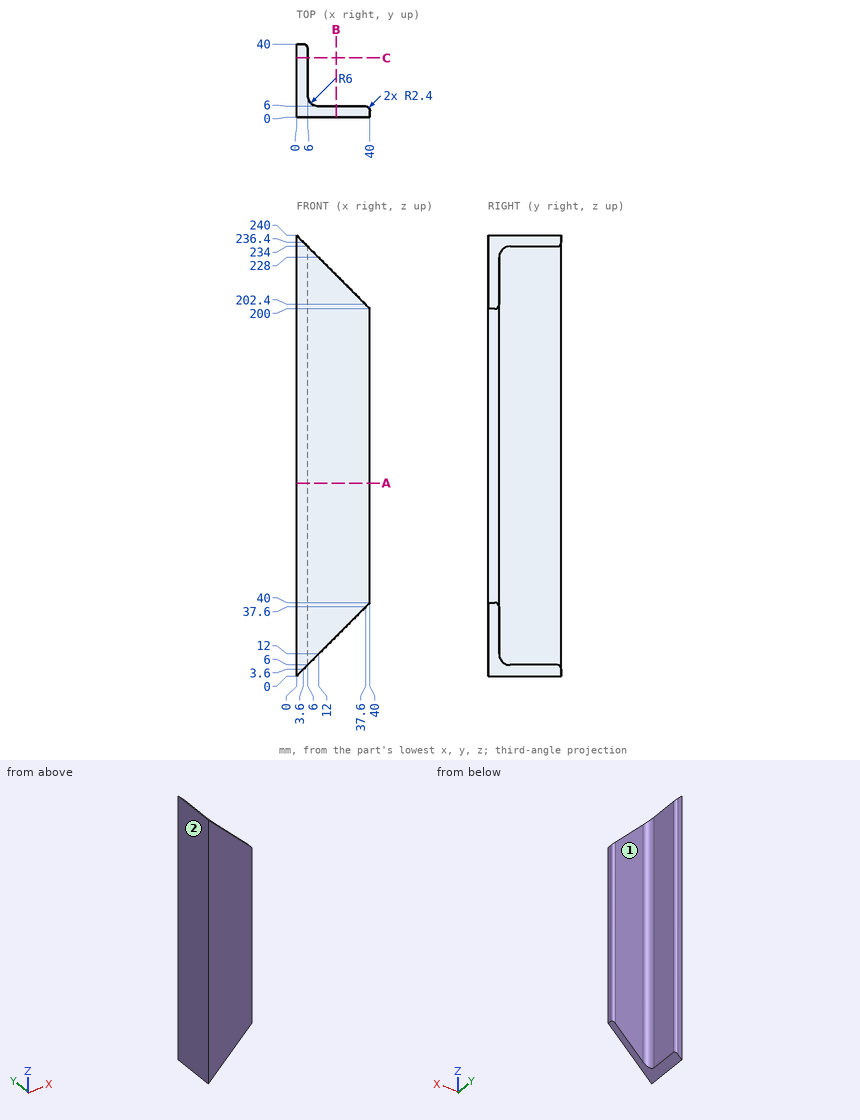
Job drawing, mm, ordinate dimensions from the low corner. One solid piece. A direction names the side the tool comes from. Coordinates: 2 decimals unless noted, no trailing zeros. Write each loop counter-clockwise with the first axis right and the second up, starting at its lowest first coordinate (ties: lowest second). Pieces come first, ordered by that corner, then holes.
Item 1: Slice it at A-A (z = 105). Write the cut outline in (x, y).
Item 2: Pin check, flat tips, straight feed: pin 1 (3 mm diameter, centred on x = 22.5, z = 57.5, fed in from +Y); pin 2 (2 mm diameter, centred on y = 35.5, z = 153, fed in from +X); pin 3 (12 mm diameter, centred on y = 10, z = 93.5, fed in from +X). Stop position of each tip, or through.
Item 3: Slice it at C-C (y = 32.5). Write the cut outline in (x, z).
Item 4: Probe line 1 (Y direction, x = 15.5, z = 143.5); line 2 (Y direction, x = 8.5, z = 120.5). List the from-to ranges inside material, lowest first.
Item 5: Slice it at B-B (x = 21.5). Write the cut outline in (y, z), and give its area (3 significant figures).
Item 6: Which spindle directions (+Z, -Z, +X, -X, +Y, -Y) get a long thin tool onto all of the face, cutting with end or side? Do the marked faces 1 and 2. Say none if no direction does.
Results found:
1. outline: (0, 0) - (40, 0) - (40, 3.6) arc R2.4 ccw to (37.6, 6) - (12, 6) arc R6 cw to (6, 12) - (6, 37.6) arc R2.4 ccw to (3.6, 40) - (0, 40) - close
2. pin 1: stops at y = 6
2. pin 2: stops at x = 6
2. pin 3: stops at x = 39.97
3. outline: (0, 0) - (6, 6) - (6, 234) - (0, 240) - close
4. line 1: y = 0 to 6
4. line 2: y = 0 to 7.13
5. outline: (0, 21.5) - (6, 21.5) - (6, 218.5) - (0, 218.5) - close
5. area: 1,180 mm2
6. face 1: +Z, -Z, +X, +Y
6. face 2: +Z, -Z, -X, +Y, -Y
